```python
from build123d import *

# Parameters (mm, degrees)
SKETCH1_R               = 10
SKETCH1_R_2             = 5
BOSS_EXTRUDE1_DEPTH     = 10
SKETCH2_R               = 17.5
BOSS_EXTRUDE2_DEPTH     = 6
SKETCH3_W               = 5
SKETCH3_H               = 3
CUT_EXTRUDE1_DEPTH      = 27
CUT_EXTRUDE1_DEPTH_BACK = 20
SKETCH4_R               = 5
CUT_EXTRUDE2_DEPTH      = 20
SKETCH6_W               = 2.522698513
SKETCH6_H               = 3
CUT_EXTRUDE3_DEPTH      = 20


with BuildPart() as part:
    # Sketch1 → Boss-Extrude1 (new body)
    with BuildSketch(Plane(origin=(0, 0, 0), x_dir=(1, 0, 0), z_dir=(0, 1, 0))):
        Circle(SKETCH1_R)
        Circle(SKETCH1_R_2, mode=Mode.SUBTRACT)
    extrude(amount=BOSS_EXTRUDE1_DEPTH)

    # Sketch2 → Boss-Extrude2 (add)
    with BuildSketch(Plane(origin=(0, 10, 0), x_dir=(1, 0, 0), z_dir=(0, 1, 0))):
        Circle(SKETCH2_R)
    extrude(amount=BOSS_EXTRUDE2_DEPTH)

    # Sketch3 → Cut-Extrude1 (cut, two sides)
    with BuildSketch(Plane.XY) as cut_extrude1_sk:
        with Locations((0, 14.5)):
            Rectangle(SKETCH3_W, SKETCH3_H)
    extrude(amount=CUT_EXTRUDE1_DEPTH, mode=Mode.SUBTRACT)
    extrude(cut_extrude1_sk.sketch, amount=-CUT_EXTRUDE1_DEPTH_BACK, mode=Mode.SUBTRACT)

    # Sketch4 → Cut-Extrude2 (cut)
    with BuildSketch(Plane.XZ.offset(-10)):
        Circle(SKETCH4_R)
    extrude(amount=-CUT_EXTRUDE2_DEPTH, mode=Mode.SUBTRACT)

    # Sketch6 → Cut-Extrude3 (cut)
    with BuildSketch(Plane.XZ):
        with Locations((5.927019422, 0)):
            Rectangle(SKETCH6_W, SKETCH6_H)
    extrude(amount=-CUT_EXTRUDE3_DEPTH, mode=Mode.SUBTRACT)


solid = part.part
```
Check sheet for the modelled part. Datum: model origin and axes. Units: mm. A direction names the side the tool comes from. Give positions to 0.01 mm unless a question says otherwise; leave off trailing zeros. Loops run counter-clockwise (first coordinate to the right, second up) from the corner with the lowest first, then second, coordinate; pieces in that order, holes last. Notation, with made-up numbers: M 63,55.5 L 104,55.5 A35 cw 104,87.5 Z; hole C 54,26 d2. An arc over 180 degrees is marked long. Answer in a Markdown table with one row per item.
1) Thickness scan on line 1 (Z direction, x = 0, y = 10.75); line 2 (X direction, y = 6, z = 0); line 3 (Z direction, x = 0, y = 6.75). Record the ranges inside material, lowest first.
Solutions:
| item | result |
|---|---|
| line 1 | z = -17.5 to -5, 5 to 17.5 |
| line 2 | x = -10 to -5, 7.19 to 10 |
| line 3 | z = -10 to -5, 5 to 10 |
2) Depth check by flat-ended pin: pin 1 (1.9 mm diameter, centred on x = 6.5, y = 10.5, fed in from -Z); pin 2 (3 mm diameter, centred on x = 9, y = 11.5, fed in from -Z); pin 3 (4 mm diameter, centred on y = 2, z = -8.5, fed in from +X); pin 4 (13 mm diameter, centred on x = 0, z = 0, fed in from +Y). Enter the tip coordinate at first touch or a pass-through.
Solutions:
| item | result |
|---|---|
| pin 1 | stops at z = -16.6 |
| pin 2 | stops at z = -15.81 |
| pin 3 | stops at x = 7.6 |
| pin 4 | stops at y = 16 |
3) Mould release check, pull along X, two halves, no side actions. Record for faces 1 (the face through (-2.17, 4.93, 9.76)), 2 (the face through (7.188, 8, 0)), 3 (the face through (-5, 0, 2)), 4 (the face through (-5, 8, 0)): released by +X, released by -X, zero draft, split by the parting line, or undercut.
Solutions:
| item | result |
|---|---|
| face 1 | split by the parting line |
| face 2 | undercut |
| face 3 | zero draft |
| face 4 | undercut |
4) Cross-section at C-C (y = 3.25). Enter the section's corners in (x, z), plus the area to 3 significant figures.
Solutions:
| item | result |
|---|---|
| outline | C 0,0 d20; hole M 4.77,-1.5 L 7.19,-1.5 L 7.19,1.5 L 4.77,1.5 A5 ccw long Z |
| area | 229 mm^2 |
5) Tool access check on faces 5 (the face through (8, 16, 0)), 6 (the face through (6, 8, -1.5)), 7 (the face through (2.5, 14, -11)), 8 (the face through (8, 10, 8)). Record the directions out of +Z, -Z, +X, -X, +Y, -Y that give a thin tool (end or side, any length) a straight path to the whole face; none if there is none.
Solutions:
| item | result |
|---|---|
| face 5 | +Z, -Z, +X, -X, +Y |
| face 6 | +Y, -Y |
| face 7 | +Z, -Z, +Y |
| face 8 | -Y |
6) Cross-section at B-B (z = 0). Enter the section's corners in (x, y).
Solutions:
| item | result |
|---|---|
| outline | M -17.5,10 L -10,10 L -10,0 L -5,0 L -5,16 L -17.5,16 Z; M 7.19,0 L 10,0 L 10,10 L 17.5,10 L 17.5,16 L 7.19,16 Z |
7) Cross-section at A-A (x = 0). Enter the section's corners in (y, z).
Solutions:
| item | result |
|---|---|
| outline | M 0,-10 L 10,-10 L 10,-17.5 L 13,-17.5 L 13,-5 L 0,-5 Z; M 0,5 L 13,5 L 13,17.5 L 10,17.5 L 10,10 L 0,10 Z |
8) Cross-section at D-D (z = -14). Enter the section's corners in (x, y).
Solutions:
| item | result |
|---|---|
| outline | M -10.5,10 L 10.5,10 L 10.5,16 L 2.5,16 L 2.5,13 L -2.5,13 L -2.5,16 L -10.5,16 Z |
